Design review of the part built by this model. Coordinates are the model's own, in mm. A direction names the side the tool comes from. Give positions to 0.01 mm unless a question says otherwise; leave off trailing zeros. Order: outer loops, then holes, each group sorted by start corner. A loop starts at its lowest first (then second) coordinate and runs counter-clockwise, first axis right, second up. Notation, with made-up numbers: (76, -17) -> (121, -17) arc R14 cw to (121, -12) -> close; hole circle Ø2 at (88, 52.5). An arc over 180 degrees is marked (long way). Return JSON: item names as keys, results as strings.
```python
from build123d import *

# Parameters (mm, degrees)
SKETCH1_R           = 34
BOSS_EXTRUDE1_DEPTH = 125
CHAMFER1_SIZE       = 3


with BuildPart() as part:
    # Sketch1 → Boss-Extrude1 (new body)
    with BuildSketch(Plane(origin=(0, 0, 0), x_dir=(1, 0, 0), z_dir=(0, 1, 0))):
        with Locations(Location((0, 0, 0), (0, 0, 270))):
            Circle(SKETCH1_R)
        with BuildLine():
            Line((31.5, 6.5), (31.5, -6.5))
            Line((31.5, -6.5), (25.690465157, -6.5))
            ThreePointArc((25.690465157, -6.5), (0, -26.5), (-25.690465157, -6.5))
            Line((-25.690465157, -6.5), (-31.5, -6.5))
            Line((-31.5, -6.5), (-31.5, 6.5))
            Line((-31.5, 6.5), (-25.690465157, 6.5))
            ThreePointArc((-25.690465157, 6.5), (0, 26.5), (25.690465157, 6.5))
            Line((25.690465157, 6.5), (31.5, 6.5))
        make_face(mode=Mode.SUBTRACT)
    extrude(amount=BOSS_EXTRUDE1_DEPTH)

    # Sketch2 → Revolve1 (revolve)
    with BuildSketch(Plane.XY):
        with BuildLine():
            Line((0, 125), (0, 195.638896549))
            add(Edge.make_bspline(
                [(0, 195.638896549), (33.497794894, 174.990797279), (34, 125)],
                knots=[0, 0, 0, 1, 1, 1], degree=2))
            Line((34, 125), (0, 125))
        make_face()
    revolve(axis=Axis((0, 125, 0), (0, 1, 0)))

    # Chamfer1
    # the kernel refuses this chamfer: 3 mm, written as the material it takes off along each edge
    with BuildSketch(Plane(origin=(0, 0, 0), x_dir=(0, 0, 1), z_dir=(-1, 0, 0))) as chamfer1_piece_1:
        Polygon((34, CHAMFER1_SIZE), (34 - CHAMFER1_SIZE, 0), (34, 0), align=None)
    revolve(axis=Axis((0, 0, 0), (0, 1, 0)), mode=Mode.SUBTRACT)


solid = part.part
```
Item 1: Wall thickness on L1, parallel to Z at x = 0, y = 22; L2, parallel to Z at x = 27.5, y = 15; L3, parallel to X at y = 31.5, z = 8: over which ranges is each line inside the solid? List them lowest first. Write a range as [from, to].
Result set:
{"L1": "z = [-34, -26.5], [26.5, 34]", "L2": "z = [-19.99, -6.5], [6.5, 19.99]", "L3": "x = [-33.05, -25.26], [25.26, 33.05]"}
Item 2: Machinability: for faces 5 (the face through (-0.491, 61.625, -26.495)), 6 (the face through (0, 0, -27)), which of the approach directions +Z, -Z, +X, -X, +Y, -Y give a long, thin tool a straight path to every point of the face, cutting with its end or side? Answer none if there is none.
Result set:
{"face 5": "-Y", "face 6": "+Z, -Z, +X, -X, -Y"}
Item 3: Add section A-A (y = 71). Give the boundary of the cut face in (x, z), plus the area to 3 significant figures.
Result set:
{"outline": "circle Ø68 at (0, 0); hole (-31.5, -6.5) -> (-25.69, -6.5) arc R26.5 ccw to (25.69, -6.5) -> (31.5, -6.5) -> (31.5, 6.5) -> (25.69, 6.5) arc R26.5 ccw to (-25.69, 6.5) -> (-31.5, 6.5) -> close", "area": "1,290 mm^2"}
Item 4: For pin 1 (3 mm diameter, centred on x = -28.5, y = 76, fed in from -Z); pin 2 (4.5 mm diameter, centred on x = 28, y = 89.5, fed in from +Z); pin 3 (3 mm diameter, centred on y = 38.5, z = 10, fed in from +X), all flat-tipped, find the tip position at first contact; note any pin that passes through.
Result set:
{"pin 1": "stops at z = -20.66", "pin 2": "stops at z = 22.2", "pin 3": "stops at x = 32.92"}
Item 5: Mouldability with a two-part tool opening along Z and no side actions: class faces 1 (the face through (-31.5, 62, 0)), 2 (the face through (-2, 0, 27)), 3 (the face through (31.5, 62, 0)), 4 (the face through (33.71, 63.15, -4.43)) as released by +Z, released by -Z, zero draft, split by the parting line, or undercut.
Result set:
{"face 1": "undercut", "face 2": "zero draft", "face 3": "undercut", "face 4": "split by the parting line"}
